```python
from build123d import *

# Parameters (mm, degrees)
SKETCH1_W           = 25.4
SKETCH1_H           = 25.4
SKETCH1_W_2         = 19.05
SKETCH1_H_2         = 19.05
BOSS_EXTRUDE1_DEPTH = 923.8
SKETCH2_R           = 5.175
CUT_EXTRUDE1_DEPTH  = 26.4
SKETCH3_R           = 3.675
CUT_EXTRUDE2_DEPTH  = 26.4


with BuildPart() as part:
    # Sketch1 → Boss-Extrude1 (new body)
    with BuildSketch(Plane.XY):
        Rectangle(SKETCH1_W, SKETCH1_H)
        Rectangle(SKETCH1_W_2, SKETCH1_H_2, mode=Mode.SUBTRACT)
    extrude(amount=BOSS_EXTRUDE1_DEPTH)

    # Sketch2 → Cut-Extrude1 (cut, through all)
    with BuildSketch(Plane(origin=(0, 12.7, 0), x_dir=(1, 0, 0), z_dir=(0, 1, 0))):
        with Locations((0, -100)):
            Circle(SKETCH2_R)
        with Locations((0, -200)):
            Circle(SKETCH2_R)
        with Locations((0, -300)):
            Circle(SKETCH2_R)
        with Locations((0, -400)):
            Circle(SKETCH2_R)
        with Locations((0, -500)):
            Circle(SKETCH2_R)
        with Locations((0, -600)):
            Circle(SKETCH2_R)
        with Locations((0, -700)):
            Circle(SKETCH2_R)
        with Locations((0, -800)):
            Circle(SKETCH2_R)
        with Locations((0, -900)):
            Circle(SKETCH2_R)
    extrude(amount=-CUT_EXTRUDE1_DEPTH, mode=Mode.SUBTRACT)

    # Sketch3 → Cut-Extrude2 (cut, through all)
    with BuildSketch(Plane.ZY.offset(12.7)):
        with Locations((100, 0)):
            Circle(SKETCH3_R)
        with Locations((200, 0)):
            Circle(SKETCH3_R)
        with Locations((300, 0)):
            Circle(SKETCH3_R)
    extrude(amount=-CUT_EXTRUDE2_DEPTH, mode=Mode.SUBTRACT)


solid = part.part
```
Read the model definition and answer for the solid it produces. Units are mm, in the model's axes. A direction names the side the tool comes from. Give positions to 0.01 mm unless a question says otherwise; leave off trailing zeros. Write each loop counter-clockwise with the first axis right and the second up, starting at its lowest first coordinate (ties: lowest second). Pieces come first, ordered by that corner, then holes. Notation, with made-up numbers: (27, -0.5) -> (31, -0.5) arc R21 cw to (31, 35.5) -> close; hole circle Ø6 at (0.25, 50.5). An arc over 180 degrees is marked (long way). Answer in a Markdown table with one row per item.
1) Straight lines are drawn through the part: line 1 (X direction, y = 7.25, z = 204) (3 decimals); line 2 (X direction, y = -10, z = 501). For each, find the intervals that lie inside material, in ascending order. Write a range as [from, to].
Results list:
| item | result |
|---|---|
| line 1 | [-12.7, -9.525], [9.525, 12.7] |
| line 2 | [-12.7, -5.08], [5.08, 12.7] |
2) Section A-A on z = 237.5 is taken. Give the vertices of the cut face in (x, y) (3 decimals), plus the area to 3 significant figures.
Results list:
| item | result |
|---|---|
| outline | (-12.7, -12.7) -> (12.7, -12.7) -> (12.7, 12.7) -> (-12.7, 12.7) -> close; hole (-9.525, -9.525) -> (9.525, -9.525) -> (9.525, 9.525) -> (-9.525, 9.525) -> close |
| area | 282 mm^2 |
3) Section B-B on x = 0 is taken. Count the separate pieces of the cut face and the enclosed holes in it, plus the area to 3 significant figures.
Results list:
| item | result |
|---|---|
| separate pieces | 20 |
| enclosed holes | 0 |
| area | 5,270 mm^2 |
4) Determine the mould class of faces 3 (the flat face through (-9.525, 0, 455)), 4 (the flat face through (11, 0, 0)), 5 (the flat face through (12.7, 0, 455)) for opening direction X: released by +X, released by -X, zero draft, split by the parting line, or undercut.
Results list:
| item | result |
|---|---|
| face 3 | undercut |
| face 4 | zero draft |
| face 5 | released by +X |
5) A tool of negligible diameter and unlimited length cuts with its end or side. For faces 1 (the flat face through (0, 9.525, 455)), 2 (the flat face through (0, 12.7, 455)), from which of +Z, -Z, +X, -X, +Y, -Y can it reach the whole face along a straight path? Write none if from no direction.
Results list:
| item | result |
|---|---|
| face 1 | +Z, -Z |
| face 2 | +Z, -Z, +X, -X, +Y |
